from build123d import *

# Parameters (mm, degrees)
F1_DEPTH = 12.7
F3_DEPTH = 6.35
F4_R     = 2.54


with BuildPart() as f1:
    # F0 (on Front) → F1 (new body)
    with BuildSketch(Plane.XZ):
        with BuildLine():
            Line((-8.89, 0), (-8.89, 35.995271902))
            ThreePointArc((-8.89, 35.995271902), (-21.2029287752, 30.4159088415), (-30.6973562447, 20.7933647802))
            ThreePointArc((-30.6973562447, 20.7933647802), (-10.8749915983, -35.4461035522), (37.0768350766, 0))
            ThreePointArc((37.0768350766, 0), (35.3625750984, 11.1436072124), (30.3783139408, 21.256757547))
            Line((30.3783139408, 21.256757547), (8.89, 35.995271902))
            ThreePointArc((8.89, 35.995271902), (8.8799379581, 35.9977555017), (8.8698752224, 36.0002362886))
            Line((8.8698752224, 36.0002362886), (8.8698752224, 0))
            Line((8.8698752224, 0), (-8.89, 0))
        make_face()
        with BuildLine():
            ThreePointArc((-30.6973562447, 20.7933647802), (-21.2029287752, 30.4159088415), (-8.89, 35.995271902))
            Line((-8.89, 35.995271902), (-8.89, 45.0685620308))
            Line((-8.89, 45.0685620308), (-8.89, 65.0674526496))
            Line((-8.89, 65.0674526496), (-30.6973562447, 20.7933647802))
        make_face()
        with BuildLine():
            Line((-8.89, 45.0685620308), (-8.89, 35.995271902))
            ThreePointArc((-8.89, 35.995271902), (-0.010364022, 37.0768336281), (8.8698752224, 36.0002362886))
            Line((8.8698752224, 36.0002362886), (8.8698752224, 45.0685620308))
            Line((8.8698752224, 45.0685620308), (-8.89, 45.0685620308))
        make_face()
        with BuildLine():
            ThreePointArc((8.8698752224, 36.0002362886), (-0.010364022, 37.0768336281), (-8.89, 35.995271902))
            Line((-8.89, 35.995271902), (-8.89, 0))
            Line((-8.89, 0), (8.8698752224, 0))
            Line((8.8698752224, 0), (8.8698752224, 36.0002362886))
        make_face()
        with BuildLine():
            Line((8.89, 65.0674526496), (8.89, 35.995271902))
            ThreePointArc((8.89, 35.995271902), (20.9715538596, 30.5758994636), (30.3783139408, 21.256757547))
            Line((30.3783139408, 21.256757547), (31.053926761, 20.7933647802))
            Line((31.053926761, 20.7933647802), (8.89, 65.0674526496))
        make_face()
        with BuildLine():
            ThreePointArc((30.3783139408, 21.256757547), (20.9715538596, 30.5758994636), (8.89, 35.995271902))
            Line((8.89, 35.995271902), (30.3783139408, 21.256757547))
        make_face()
    extrude(amount=F1_DEPTH)

    # F2 (on face) → F3 (join)
    with BuildSketch(Plane.XZ.offset(12.7)):
        with BuildLine():
            Line((8.3370473279, -3.6677770405), (9.1081802006, 0))
            ThreePointArc((9.1081802006, 0), (-8.9133124025, 1.8739820121), (8.3370473279, -3.6677770405))
        make_face()
        with BuildLine():
            ThreePointArc((8.3370473279, -3.6677770405), (8.9133124025, -1.8739820121), (9.1081802006, 0))
            Line((9.1081802006, 0), (8.3370473279, -3.6677770405))
        make_face()
        Polygon((27.6729999866, 27.547016816), (5.6928377599, 14.1950091347), (12.3025802895, 6.641021464), (35.9087884426, 20.7933647802), align=None)
        Polygon((26.466306299, 37.8012210131), (27.6729999866, 27.547016816), (35.9087884426, 20.7933647802), (35.9087884426, 37.8012210131), (32.9793743131, 43.6529430466), (26.466306299, 42.9304087149), align=None)
    extrude(amount=F3_DEPTH)

    # F4
    f4_edges = [f1.edges().sort_by_distance(p)[0] for p in [
        (-8.337047, -19.05, 3.667777),
    ]]
    fillet(f4_edges, radius=F4_R)


solid = f1.part
Design review of the part built by this model. Coordinates are the model's own, in mm. A direction names the side the tool comes from. Give positions to 0.01 mm unless a question says otherwise; leave off trailing zeros. Write each loop counter-clockwise with the first axis right and the second up, starting at its lowest first coordinate (ties: lowest second). Pieces come first, ordered by that corner, then holes. Notation, with made-up numbers: M 59,1 L 96,1 A30 cw 96,34 Z; hole C -14.5,85.25 d2. An arc over 180 degrees is marked long. Answer as a JSON object with one key per item and string values. Group by question number.
1) We need section D-D (z = 47.5). Give the boundary of the cut face in (x, y).
2) Clearance check with flat-ended pins moving along their axes: pin 1 Ø4 at (y, z) = (-11, 7) entering from +X; pin 2 Ø5 at (y, z) = (-15, 28) entering from +X; pin 3 Ø8 at (x, y) = (4, -3.5) entering from -Z. State where each tip first meets the part, or that it passes through.
3) Tool access review of faces 4 (the face through (8.95, -15.83, 10.47)), 5 (the face through (26.466, -16, 40)), 6 (the face through (23.94, -15.83, 13.62)), 7 (the face through (0, -6, 45.069)): name each direction out of +Z, -Z, +X, -X, +Y, -Y from which nothing blocks a thin tool from reaching the whole face with its end or side.
4) Mouldability with a two-part tool opening along Z and no side actions: class faces 1 (the face through (29.8, -15.8, 43.3)), 2 (the face through (27.06, -15.83, 32.75)), 3 (the face through (-8.89, -6, 55)) as released by +Z, released by -Z, zero draft, split by the parting line, or undercut.
5) We need section C-C (x = 18.5). Give the boundary of the cut face in (y, z), and give its area (3 significant figures).
6) We need section A-A (y = -14.25). Give the boundary of the cut face in (x, z) (3 decimals), and give its area (3 significant figures).
7) For line 1 along Y through (x, z) = (9, -6.5); line 2 along Y through (x, z) = (30.5, 32); line 3 along Z through (x, y) = (-2, -12), list the stretches that pass through material, from the lowest coordinate up.
8) We need section B-B (z = 33). Give the boundary of the cut face in (x, y), and give its area (3 significant figures).
Answer key:
{
 "1": {"outline": "M -17.54,-12.7 L -8.89,-12.7 L -8.89,0 L -17.54,0 Z; M 8.89,-12.7 L 17.68,-12.7 L 17.68,0 L 8.89,0 Z"},
 "2": {"pin 1": "stops at x = 36.74", "pin 2": "stops at x = 35.91", "pin 3": "stops at z = -37.08"},
 "3": {"face 4": "-Y", "face 5": "+Z, -X, +Y, -Y", "face 6": "-Z, +X, -Y", "face 7": "+Z, +Y, -Y"},
 "4": {"face 1": "released by +Z", "face 2": "undercut", "face 3": "zero draft"},
 "5": {"outline": "M -19.05,10.36 L -12.7,10.36 L -12.7,-32.13 L 0,-32.13 L 0,45.87 L -12.7,45.87 L -12.7,21.97 L -19.05,21.97 Z", "area": "1,060 mm²"},
 "6": {"outline": "C 0,0 d18.216; M 5.693,14.195 L 12.303,6.641 L 35.909,20.793 L 35.909,37.801 L 32.979,43.653 L 26.466,42.93 L 26.466,37.801 L 27.673,27.547 Z", "area": "689 mm²"},
 "7": {"line 1": "y = -12.7 to 0", "line 2": "y = -19.05 to -12.7", "line 3": "z = -37.02 to 45.07"},
 "8": {"outline": "M -24.68,-12.7 L 24.94,-12.7 L 24.94,0 L -24.68,0 Z; M 27.03,-19.05 L 35.91,-19.05 L 35.91,-12.7 L 27.03,-12.7 Z", "area": "687 mm²"}
}
